Verification items for the finished model (mm, model axes). Face numbers are marked on the shaded views. A direction names the side the tool comes from. Give positions to 0.01 mm unless a question says otherwise; leave off trailing zeros. Loops run counter-clockwise (first coordinate to the right, second up) from the corner with the lowest first, then second, coordinate; pieces in that order, holes last. Notation, with made-up numbers: (-29, 77) -> (21, 77) arc R22 ccw to (21, 104) -> close; hole circle Ø3 at (17.25, 24.5). An arc over 180 degrees is marked (long way). Answer in a Markdown table with one row per item. Add a question column.
Q1. Section check C-C on z = 7.5. Enter the section's corners in (x, y).
Q2. Section check A-A on x = 0. Enter the section's corners in (y, z), and give its area (4 significant figures).
Q3. Gauge pin test, flat ends, axial feed: P1, Ø1.6, axis at x = -5, y = 3, coming from the +Z side; P2, Ø1, axis at y = 5, z = -6.5, coming from the -X side; P3, Ø6.5, axis at x = 24.5, z = 5, coming from the +Y side. Record the tip position at first contact, or that the pin passes through.
Q4. Release check for a two-part mould opening along X. For the marked faces 3, 4 and 5 record: pulls with the +X half, pulls with the -X half, needs draft (parallel to the pull), parting line crosses it, or undercut.
Q5. Section check B-B on y = 6. Enter the section's corners in (x, z) (3 decimals).
Q6. Section check D-D on y = 3.7. Enter the section's corners in (x, z) (3 decimals), and give its area (3 significant figures).
Q7. Material ranges on probe 1 along X at (y, z) = (1.75, 0.5); probe 2 along Y at (x, z) = (-9.3, 0); probe 3 along Y at (x, z) = (13.5, 3.25), recorded low to high.
Q8. Set-up check for the marked faces 1 and 2: record each of +Z, -Z, +X, -X, +Y, -Y from which the full face is reachable in a straight line by a thin tool's end or side.
```python
from build123d import *

# Parameters (mm, degrees)
EXTRUDE_1_DEPTH       = 3
SKETCH_4_R            = 11
EXTRUDE_2_DEPTH       = 4.5
SKETCH_5_R            = 4.1
SKETCH_5_R_2          = 1.55
CUT_EXTRUDE_1_DEPTH   = 8.5
SKETCH_7_W            = 5.6
SKETCH_7_H            = 5.6
CUT_EXTRUDE_812_DEPTH = 2.1
SKETCH_8_R            = 1.55
CUT_EXTRUDE_M3_DEPTH  = 7.9


with BuildPart() as part:
    # 草图2 → 凸台-拉伸1 (new body)
    with BuildSketch(Plane(origin=(0, 0, 0), x_dir=(1, 0, 0), z_dir=(0, 1, 0))):
        with BuildLine():
            Line((1.924560376, 10.830330898), (35.874800171, 4.797340137))
            ThreePointArc((35.874800171, 4.797340137), (39.999967838, -0.143471364), (35.839463489, -5.054563924))
            Line((35.839463489, -5.054563924), (1.846819677, -10.843858035))
            ThreePointArc((1.846819677, -10.843858035), (-10.999929243, 0.039454403), (1.924560376, 10.830330898))
        make_face()
    extrude(amount=EXTRUDE_1_DEPTH)

    # 草图4 → 凸台-拉伸2 (add)
    with BuildSketch(Plane(origin=(0, 3, 0), x_dir=(1, 0, 0), z_dir=(0, 1, 0))):
        Circle(SKETCH_4_R)
    extrude(amount=EXTRUDE_2_DEPTH)

    # 草图5 → 切除-拉伸1 (cut, through all)
    with BuildSketch(Plane.XZ):
        Circle(SKETCH_5_R)
        with Locations((35, 0.125537544)):
            Circle(SKETCH_5_R_2)
    extrude(amount=-CUT_EXTRUDE_1_DEPTH, mode=Mode.SUBTRACT)

    # 草图7 → Cut-Extrude 812 (cut, symmetric)
    with BuildSketch(Plane(origin=(-4.1, 0, 0), x_dir=(0, 0, -1), z_dir=(1, 0, 0))):
        with Locations((0, 3.7)):
            Rectangle(SKETCH_7_W, SKETCH_7_H)
    extrude(amount=CUT_EXTRUDE_812_DEPTH, both=True, mode=Mode.SUBTRACT)

    # 草图8 → 切除-M3孔 (cut, through all)
    with BuildSketch(Plane(origin=(-4.1, 0, 0), x_dir=(0, 0, -1), z_dir=(1, 0, 0))):
        with Locations((0, 3.7)):
            Circle(SKETCH_8_R)
    extrude(amount=-CUT_EXTRUDE_M3_DEPTH, mode=Mode.SUBTRACT)


solid = part.part
```
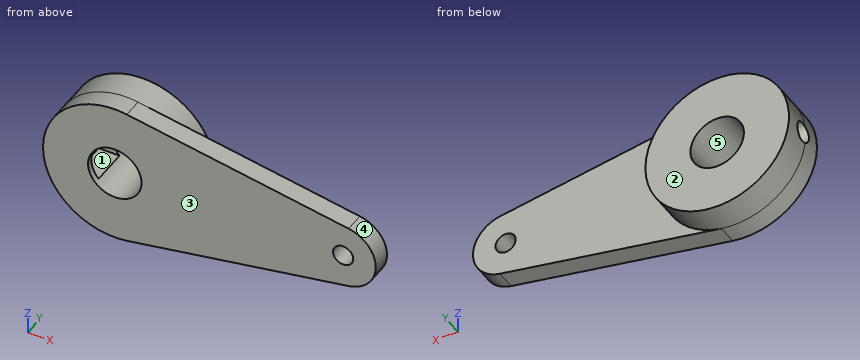
Taken from the geometry:
| question | item | result |
|---|---|---|
| 1 | outline | (-8.05, 0) -> (21.48, 0) -> (21.48, 3) -> (8.05, 3) -> (8.05, 7.5) -> (-8.05, 7.5) -> close |
| 2 | outline | (0, -11) -> (7.5, -11) -> (7.5, -4.1) -> (0, -4.1) -> close; (0, 4.1) -> (7.5, 4.1) -> (7.5, 11) -> (0, 11) -> close |
| 2 | area | 103.5 mm² |
| 3 | P1 | stops at z = 10.17 |
| 3 | P2 | stops at x = -9.22 |
| 3 | P3 | stops at y = 3 |
| 4 | face 3 | needs draft |
| 4 | face 4 | pulls with the +X half |
| 4 | face 5 | undercut |
| 5 | outline | circle Ø22 at (0, 0); hole (-6.2, -2.8) -> (-2.995, -2.8) arc R4.1 ccw (long way) to (-2.995, 2.8) -> (-6.2, 2.8) -> close |
| 6 | outline | (-10.89, -1.55) arc R11 ccw (long way) to (-10.89, 1.55) -> (-6.2, 1.55) -> (-6.2, 2.8) -> (-2.995, 2.8) arc R4.1 cw (long way) to (-2.995, -2.8) -> (-6.2, -2.8) -> (-6.2, -1.55) -> close |
| 6 | area | 299 mm² |
| 7 | probe 1 | x = -10.99 to -6.2, 4.07 to 33.5, 36.5 to 39.99 |
| 7 | probe 2 | y = 0 to 2.15, 5.25 to 7.5 |
| 7 | probe 3 | y = 0 to 3 |
| 8 | face 1 | none |
| 8 | face 2 | +Z, -Z, +X, -X, +Y |
